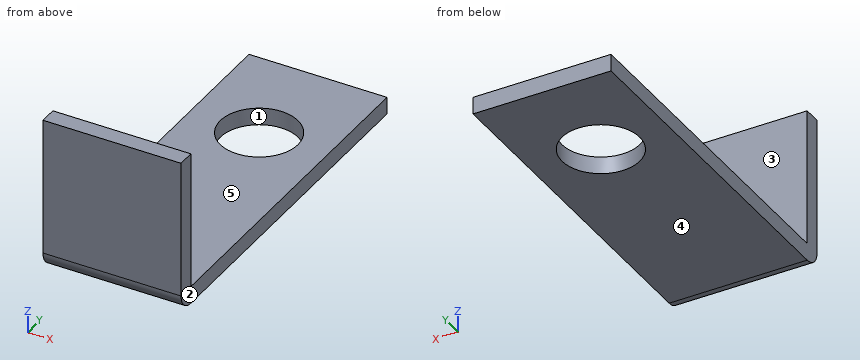
from build123d import *

# Parameters (mm, degrees)
SKETCH1_W           = 25.4
SKETCH1_H           = 63.5
BOSS_EXTRUDE1_DEPTH = 3.175
SKETCH2_W           = 25.4
SKETCH2_H           = 3.175
BOSS_EXTRUDE2_DEPTH = 25.4
BOSS_EXTRUDE3_DEPTH = 25.4
SKETCH4_R           = 7.14375
CUT_EXTRUDE1_DEPTH  = 4.175


with BuildPart() as part:
    # Sketch1 → Boss-Extrude1 (new body)
    with BuildSketch(Plane.XY):
        Rectangle(SKETCH1_W, SKETCH1_H)
    extrude(amount=BOSS_EXTRUDE1_DEPTH)



with BuildPart() as body_2:
    # Sketch2 → Boss-Extrude2 (new body)
    with BuildSketch(Plane(origin=(12.7, 0, 0), x_dir=(0, 0, -1), z_dir=(1, 0, 0))):
        with Locations((-15.875, -33.3375)):
            Rectangle(SKETCH2_W, SKETCH2_H)
    extrude(amount=-BOSS_EXTRUDE2_DEPTH)


with BuildPart() as part_1:
    add(part.part)

    add(body_2.part)  # Boss-Extrude3 merges body 2
    # Sketch3 → Boss-Extrude3 (add)
    with BuildSketch(Plane(origin=(12.7, 0, 0), x_dir=(0, 0, -1), z_dir=(1, 0, 0))):
        with BuildLine():
            Line((0, -31.75), (-3.175, -31.75))
            Line((-3.175, -31.75), (-3.175, -34.925))
            ThreePointArc((-3.175, -34.925), (-0.92993597, -33.99506403), (0, -31.75))
        make_face()
    extrude(amount=-BOSS_EXTRUDE3_DEPTH)

    # Sketch4 → Cut-Extrude1 (cut, through all)
    with BuildSketch(Plane.XY.offset(3.175)):
        with Locations((0, 12.7)):
            Circle(SKETCH4_R)
    extrude(amount=-CUT_EXTRUDE1_DEPTH, mode=Mode.SUBTRACT)


solid = part_1.part
The listing builds one solid part. Answer for the finished solid, in the listing's coordinates (mm). Face numbers are marked on the shaded views. A direction names the side the tool comes from. Round coordinates to 2 decimals unless told otherwise and drop trailing zeros. Write each loop counter-clockwise with the first axis right and the second up, starting at its lowest first coordinate (ties: lowest second). Pieces come first, ordered by that corner, then holes. Notation, with made-up numbers: (11.25, 42.25) - (40.25, 42.25) arc R12 ccw to (40.25, 62.25) - close; hole circle Ø2 at (66.5, -10.5). An arc over 180 degrees is marked (long way). Use one line per item in the form item = value. Start each with the question number.
Item 1: A cutting plane is placed at A-A (y = 12.7). Write down the section's boundary in (x, z) (3 decimals), plus the area to 3 significant figures.
Item 2: A tool of negligible diameter and unlimited length cuts with its end or side. For the marked faces 4 and 5, from which of +Z, -Z, +X, -X, +Y, -Y can it reach the whole face along a straight path? Write none if from no direction.
Item 3: Find the intervals of material crossed by line 1 (Z direction, x = -2.5, y = -24.5) (3 decimals); line 2 (Y direction, x = 10.5, z = 13.5) (3 decimals); line 3 (Y direction, x = 0, z = 1.1), in increasing order. Write a range as [from, to].
Item 4: A cutting plane is placed at C-C (z = 21). Write down the section's boundary in (x, y) (3 decimals).
Item 5: A cutting plane is placed at D-D (z = 2.5). Write down the section's boundary in (x, y), plus the area to 3 significant figures.
Item 6: Flat-ended cylindrical pins translate along their axes: pin 1 Ø10 at (x, z) = (-3.5, 23.5) entering from +Y; pin 2 Ø3 at (x, y) = (-8.5, -18) entering from +Z (3 decimals). Find the tip coordinate at first contact, or state that the pin passes through.
Item 7: Determine the mould class of the marked faces 1, 2 and 3 for opening direction X: +X half, -X half, draft (parallel to the pull), parting line (faces both ways), or undercut.
Item 8: A cutting plane is placed at B-B (x = 0). Write down the section's boundary in (y, z) (3 decimals).
The answers:
q1.outline = (-12.7, 0) - (-7.144, 0) - (-7.144, 3.175) - (-12.7, 3.175) - close; (7.144, 0) - (12.7, 0) - (12.7, 3.175) - (7.144, 3.175) - close
q1.area = 35.3 mm^2
q2.face_4 = -Z, +X, -X, +Y, -Y
q2.face_5 = +Z, +X, -X, +Y
q3.line_1 = [0, 3.175]
q3.line_2 = [-34.925, -31.75]
q3.line_3 = [-34.15, 5.56], [19.84, 31.75]
q4.outline = (-12.7, -34.925) - (12.7, -34.925) - (12.7, -31.75) - (-12.7, -31.75) - close
q5.outline = (-12.7, -34.85) - (12.7, -34.85) - (12.7, 31.75) - (-12.7, 31.75) - close; hole circle Ø14.29 at (0, 12.7)
q5.area = 1,530 mm^2
q6.pin_1 = -31.75
q6.pin_2 = 3.175
q7.face_1 = undercut
q7.face_2 = +X half
q7.face_3 = draft
q8.outline = (-34.925, 3.175) arc R3.175 ccw to (-31.75, 0) - (5.556, 0) - (5.556, 3.175) - (-31.75, 3.175) - (-31.75, 28.575) - (-34.925, 28.575) - close; (19.844, 0) - (31.75, 0) - (31.75, 3.175) - (19.844, 3.175) - close
